Geometry check sheet. Reference: drawing and pictorial views, mm from the part's lowest x, y, z. A direction names the side the tool comes from. Give positions to 0.01 mm unless a question says otherwise; leave off trailing zeros. Write each loop counter-clockwise with the first axis right and the second up, starting at its lowest first coordinate (ties: lowest second). Pieces come first, ordered by that corner, then holes. Notation, with made-up numbers: M -37,-22 L 2,-22 A8 ccw 2,-12 Z; hole C 39.5,45.5 d5. An arc over 180 degrees is marked long. Answer as a JSON object with one key per item and string values.
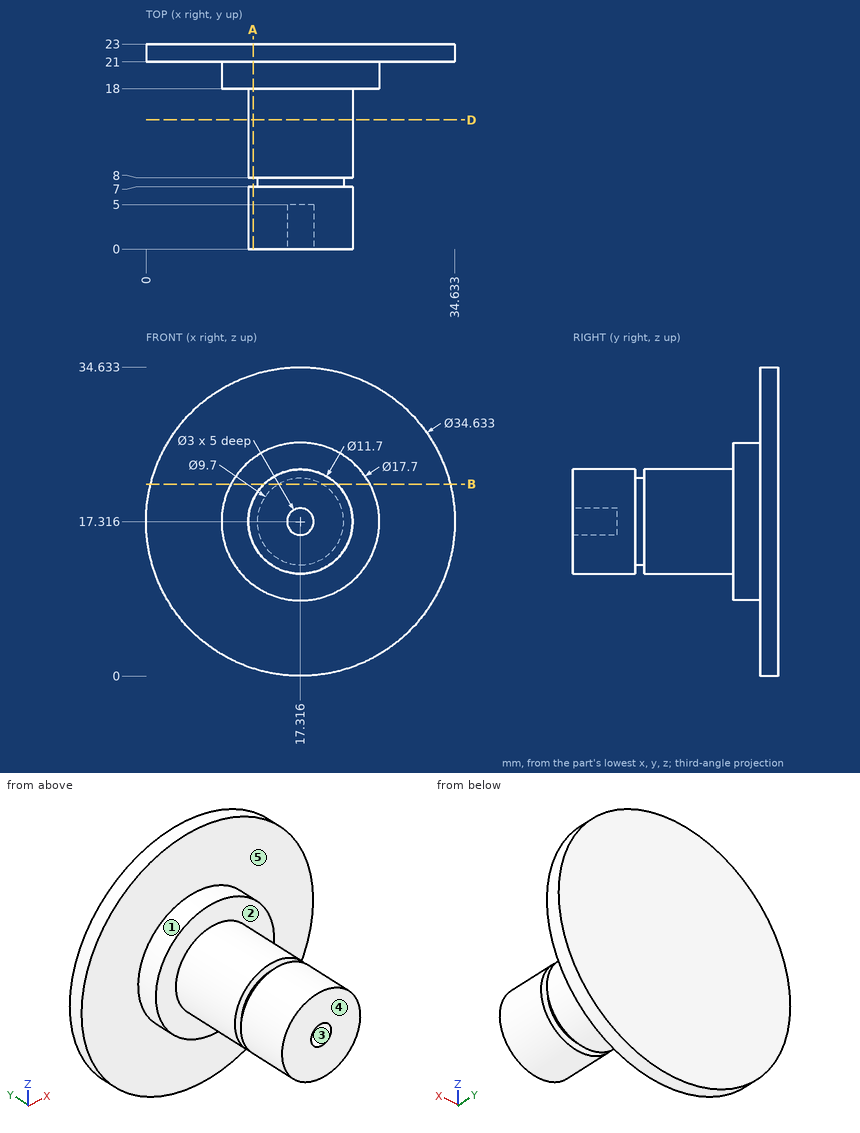
1) Section check A-A on x = 12. Record the boundary of the cut face in (y, z) (1 decimal).
Completed:
{"outline": "M 0,14.9 L 7,14.9 L 7,19.8 L 0,19.8 Z; M 8,14.9 L 18,14.9 L 18,10.2 L 21,10.2 L 21,0.8 L 23,0.8 L 23,33.8 L 21,33.8 L 21,24.4 L 18,24.4 L 18,19.8 L 8,19.8 Z"}
2) Section check D-D on y = 14.5. Record the boundary of the cut face in (x, z).
Completed:
{"outline": "C 17.32,17.32 d11.7"}
3) Thickness scan on L1, parallel to Y at x = 21.5, z = 26; L2, parallel to Y at x = 16.5, z = 25; L3, parallel to Z at x = 15, y = 9 (1 decimal). Record the ranges inside material, lowest first.
Completed:
{"L1": "y = 21 to 23", "L2": "y = 18 to 23", "L3": "z = 11.9 to 22.7"}
4) Release check for a two-part mould opening along Z. For the marked faces 1, 2 and 3 record: pulls with the +Z half, pulls with the -Z half, needs draft (parallel to the pull), parting line crosses it, or undercut.
Completed:
{"face 1": "parting line crosses it", "face 2": "needs draft", "face 3": "undercut"}
5) Section check B-B on z = 21.5. Record the boundary of the cut face in (x, y) (1 decimal).
Completed:
{"outline": "M 0.5,21 L 9.5,21 L 9.5,18 L 13.2,18 L 13.2,8 L 14.9,8 L 14.9,7 L 13.2,7 L 13.2,0 L 21.4,0 L 21.4,7 L 19.8,7 L 19.8,8 L 21.4,8 L 21.4,18 L 25.1,18 L 25.1,21 L 34.1,21 L 34.1,23 L 0.5,23 Z"}
6) Go/stop test with flat-tipped pins: pin 1 (8 mm diameter, centred on y = 2.5, z = 20, fed in from +X); pin 2 (12 mm diameter, centred on x = 21, y = 4.5, fed in from +Z); pin 3 (1 mm diameter, centred on y = 20, z = 9.5, fed in from +X) (1 decimal). Record where each tip stops, or that it passes through.
Completed:
{"pin 1": "stops at x = 23.17", "pin 2": "stops at z = 23.17", "pin 3": "stops at x = 22.3"}
7) Access from +Z, -Z, +X, -X, +Y, -Y to the whole of each face (thin tool, end or side, straight path). Record for the marked faces 4 and 5.
Completed:
{"face 4": "+Z, -Z, +X, -X, -Y", "face 5": "-Y"}
